from build123d import *

# Parameters (mm, degrees)
SKETCH2_W               = 80
SKETCH2_H               = 44
BOSS_EXTRUDE1_DEPTH     = 3.3
FILLET1_R               = 5
SKETCH3_R               = 1.75
CUT_EXTRUDE1_DEPTH      = 46.76996832
MIRROR2_COPY_1_SKETCH_R = 1.75
MIRROR2_COPY_1_DEPTH    = 46.76996832
BOSS_EXTRUDE2_DEPTH     = 21.75
FILLET2_R               = 5
CUT_EXTRUDE2_DEPTH      = 73.174242058
BOSS_EXTRUDE3_START     = -5.75
SKETCH10_R              = 0.5
BOSS_EXTRUDE3_DEPTH     = 2
BOSS_EXTRUDE4_DEPTH     = 1
BOSS_EXTRUDE5_DEPTH     = 1
SKETCH15_R              = 2.032
CUT_EXTRUDE3_DEPTH      = 7.5


with BuildPart() as part:
    # Sketch2 → Boss-Extrude1 (new body)
    with BuildSketch(Plane(origin=(0, 0, 0), x_dir=(1, 0, 0), z_dir=(0, 1, 0))):
        Rectangle(SKETCH2_W, SKETCH2_H)
    extrude(amount=BOSS_EXTRUDE1_DEPTH)

    # Fillet1
    fillet1_edges = [part.edges().sort_by_distance(p)[0] for p in [
        (40, 1.65, 22),
        (-40, 1.65, 22),
        (-40, 1.65, -22),
        (40, 1.65, -22),
    ]]
    fillet(fillet1_edges, radius=FILLET1_R)

    # Sketch3 → Cut-Extrude1 (cut, through all)
    with BuildSketch(Plane(origin=(0, 3.3, 0), x_dir=(1, 0, 0), z_dir=(0, 1, 0))):
        with Locations(Location((33, -15, 0), (0, 0, 270))):
            Circle(SKETCH3_R)
    cut_extrude1 = extrude(amount=-CUT_EXTRUDE1_DEPTH, mode=Mode.SUBTRACT)

    # Mirror1: Cut-Extrude1 across plane
    add(cut_extrude1.mirror(Plane.XY), mode=Mode.SUBTRACT)

    # Mirror2: Cut-Extrude1 across plane
    add(cut_extrude1.mirror(Plane(origin=(0, 0, 0), x_dir=(0, 0, 1), z_dir=(1, 0, 0))), mode=Mode.SUBTRACT)

    # Mirror2 copy 1 sketch → Mirror2 copy 1 (cut, through all)
    with BuildSketch(Plane(origin=(0, 3.3, 0), x_dir=(-1, 0, 0), z_dir=(0, 1, 0))):
        with Locations(Location((33, -15, 0), (0, 0, 270))):
            Circle(MIRROR2_COPY_1_SKETCH_R)
    extrude(amount=-MIRROR2_COPY_1_DEPTH, mode=Mode.SUBTRACT)

    # Sketch4 → Boss-Extrude2 (add, symmetric)
    with BuildSketch(Plane.XY):
        Polygon((-25.5, 3.3), (-21.1, 26.5), (25.4, 15.9), (25.4, 3.3), align=None)
    extrude(amount=BOSS_EXTRUDE2_DEPTH, both=True)

    # Fillet2
    fillet2_edges = [part.edges().sort_by_distance(p)[0] for p in [
        (25.4, 9.6, -21.75),
        (-23.3, 14.9, -21.75),
        (25.4, 9.6, 21.75),
        (-23.3, 14.9, 21.75),
    ]]
    fillet(fillet2_edges, radius=FILLET2_R)

    # Sketch9 → Cut-Extrude2 (cut, through all)
    with BuildSketch(Plane(origin=(-25.218766141, 4.78286944, 0), x_dir=(0, 0, 1), z_dir=(-0.9824865243069563, 0.18633365116166412, 0))):
        with BuildLine():
            Line((-5.75, 22.104252855), (5.75, 22.104252855))
            ThreePointArc((5.75, 22.104252855), (0, 16.354252855), (-5.75, 22.104252855))
        make_face()
    extrude(amount=-CUT_EXTRUDE2_DEPTH, mode=Mode.SUBTRACT)

    # Sketch10 → Boss-Extrude3 (add)
    with BuildSketch(Plane(origin=(4.700170139, 20.618670893, 0), x_dir=(0.9749884721737534, -0.22225543666756517, 0), z_dir=(0.2222554366675652, 0.9749884721737535, 0)).offset(BOSS_EXTRUDE3_START)):
        with Locations((-16.262025835, 0)):
            Circle(SKETCH10_R)
    extrude(amount=BOSS_EXTRUDE3_DEPTH)

    # Sketch12 → Boss-Extrude4 (add, symmetric)
    with BuildSketch(Plane.XY):
        Polygon((-23.038031878, 16.281286463), (-38.252702488, 3.3), (-25.5, 3.3), align=None)
    extrude(amount=BOSS_EXTRUDE4_DEPTH, both=True)

    # Sketch14 → Boss-Extrude5 (add, symmetric)
    with BuildSketch(Plane.XY.offset(7.5)):
        Polygon((25.4, 15.243617542), (39, 3.3), (25.4, 3.3), align=None)
    boss_extrude5 = extrude(amount=BOSS_EXTRUDE5_DEPTH, both=True)

    # Mirror3: Boss-Extrude5 across plane
    add(boss_extrude5.mirror(Plane.XY))

    # Sketch15 → Cut-Extrude3 (cut)
    with BuildSketch(Plane(origin=(4.700170139, 20.618670893, 0), x_dir=(0.9749884721737534, -0.22225543666756517, 0), z_dir=(0.2222554366675652, 0.9749884721737535, 0))):
        with Locations(Location((-19.462025835, 14.75, 0), (0, 0, 180))):
            Circle(SKETCH15_R)
        with Locations(Location((14.23084575, 14.75, 0), (0, 0, 180))):
            Circle(SKETCH15_R)
    cut_extrude3 = extrude(amount=-CUT_EXTRUDE3_DEPTH, mode=Mode.SUBTRACT)

    # Mirror4: Cut-Extrude3 across plane
    add(cut_extrude3.mirror(Plane.XY), mode=Mode.SUBTRACT)


solid = part.part
Work out the finished part from the listing and answer in its coordinate system (mm). A direction names the side the tool comes from. Give positions to 0.01 mm unless a question says otherwise; leave off trailing zeros. Order: outer loops, then holes, each group sorted by start corner. A loop starts at its lowest first (then second) coordinate and runs counter-clockwise, first axis right, second up. Notation, with made-up numbers: (22, 14) -> (50, 14) arc R16 ccw to (50, 44) -> close; hole circle Ø1 at (-18.75, -4.75). An arc over 180 degrees is marked (long way). Answer as a JSON object with one key per item and string values. Group by question number.
1. Section D-D on x = -33 is taken. Determine the outline of the cut face in (y, z), plus the area to 3 significant figures.
2. Consider line 1 along Z through (x, y) = (-33, 1); line 2 along X through (y, z) = (2.35, -15); line 3 along Z through (x, y) = (16, 10.75). Determine where each line is inside the solid, lowest interval first. Write a range as [from, to].
3. Section C-C on z = 10.5 is taken. Determine the outline of the cut face in (x, y).
4. Flat-ended cylindrical pins translate along their axes: pin 1 Ø5.5 at (x, z) = (-33, 15) entering from +Y; pin 2 Ø2 at (x, z) = (33, 15) entering from -Y; pin 3 Ø14.5 at (x, y) = (-29, 8.5) entering from -Z; pin 4 Ø6.5 at (y, z) = (9.5, -2) entering from +X. Find the tip coordinate at first contact, or state that the pin passes through.
5. Section A-A on y = 2.25 is taken. Determine the outline of the cut face in (x, z), plus the area to 3 significant figures.
6. Section B-B on x = 33 is taken. Determine the outline of the cut face in (y, z), plus the area to 3 significant figures.
7. A tool of negligible diameter and unlimited length cuts with its end or side. For faces 5 (the flat face through (29, 7, -8.5)), 6 (the flat face through (26, 3.3, 0)), 7 (the flat face through (0, 12, 21.75)), from which of +Z, -Z, +X, -X, +Y, -Y can it reach the whole face along a straight path? Write none if from no direction.
8. The mould has two halves that part along X. Classify faces 1 (the cylindrical face through (-34.5, 1.7, 15.9)), 2 (the flat face through (-15.914, 17.625, 14.722)), 3 (the flat face through (32.1, 9.36, -7.51)), 4 (the flat face through (-29, 7, -1)): released by +X, released by -X, zero draft, split by the parting line, or undercut.
Result sheet:
{
 "1": {"outline": "(0, -22) -> (3.3, -22) -> (3.3, -16.75) -> (0, -16.75) -> close; (0, -13.25) -> (3.3, -13.25) -> (3.3, -1) -> (7.78, -1) -> (7.78, 1) -> (3.3, 1) -> (3.3, 13.25) -> (0, 13.25) -> close; (0, 16.75) -> (3.3, 16.75) -> (3.3, 22) -> (0, 22) -> close", "area": "131 mm^2"},
 "2": {"line 1": "z = [-22, -16.75], [-13.25, 13.25], [16.75, 22]", "line 2": "x = [-40, -34.75], [-31.25, 31.25], [34.75, 40]", "line 3": "z = [-21.75, -16.51], [-12.99, 12.99], [16.51, 21.75]"},
 "3": {"outline": "(-40, 0) -> (40, 0) -> (40, 3.3) -> (25.4, 3.3) -> (25.4, 15.9) -> (-21.1, 26.5) -> (-25.5, 3.3) -> (-40, 3.3) -> close"},
 "4": {"pin 1": "stops at y = 3.3", "pin 2": "passes through", "pin 3": "stops at z = -22", "pin 4": "stops at x = 25.4"},
 "5": {"outline": "(-40, -17) arc R5 ccw to (-35, -22) -> (35, -22) arc R5 ccw to (40, -17) -> (40, 17) arc R5 ccw to (35, 22) -> (-35, 22) arc R5 ccw to (-40, 17) -> close; hole circle Ø3.5 at (-33, -15); hole circle Ø3.5 at (-33, 15); hole circle Ø3.5 at (33, -15); hole circle Ø3.5 at (33, 15)", "area": "3,460 mm^2"},
 "6": {"outline": "(0, -22) -> (3.3, -22) -> (3.3, -16.75) -> (0, -16.75) -> close; (0, -13.25) -> (3.3, -13.25) -> (3.3, -8.5) -> (8.57, -8.5) -> (8.57, -6.5) -> (3.3, -6.5) -> (3.3, 6.5) -> (8.57, 6.5) -> (8.57, 8.5) -> (3.3, 8.5) -> (3.3, 13.25) -> (0, 13.25) -> close; (0, 16.75) -> (3.3, 16.75) -> (3.3, 22) -> (0, 22) -> close", "area": "143 mm^2"},
 "7": {"face 5": "-Z, +X, +Y", "face 6": "+Y", "face 7": "+Z, +X, -X, +Y"},
 "8": {"face 1": "undercut", "face 2": "undercut", "face 3": "released by +X", "face 4": "zero draft"}
}
